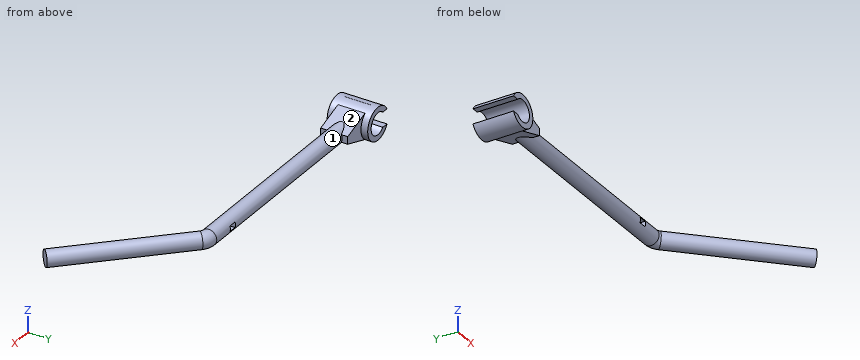
```python
from build123d import *

# Parameters (mm, degrees)
F0_R      = 6
F0_R_2    = 4
F1_DEPTH  = 7.5
F3_R      = 2.95
F4_DEPTH  = 80
F5_W      = 20
F5_H      = 5.5
F6_DEPTH  = 25
F12_DEPTH = 5
F13_W     = 3
F13_H     = 2
F14_DEPTH = 12.5
F16_R     = 2.95


with BuildPart() as f1:
    # F0 (on Front) → F1 (new body, symmetric)
    with BuildSketch(Plane.XZ):
        Circle(F0_R)
        Circle(F0_R_2, mode=Mode.SUBTRACT)
    extrude(amount=F1_DEPTH, both=True)

    # F3 (on offset) → F4 (join)
    with BuildSketch(Plane.YZ.offset(4.5)):
        Circle(F3_R)
    extrude(amount=F4_DEPTH)

    # F5 (on face) → F6 (cut)
    with BuildSketch(Plane.XZ.offset(7.5)):
        with Locations((-10, 0)):
            Rectangle(F5_W, F5_H)
    extrude(amount=-F6_DEPTH, mode=Mode.SUBTRACT)

    # F11 (on face) → F12 (join, symmetric)
    with BuildSketch(Plane.XZ):
        Polygon((13.7702096254, 1.3738754205), (0, 6.0186968185), (5.8568101376, 0), (0, -5.9087458067), (13.7702096254, -1.3786113122), align=None)
    extrude(amount=F12_DEPTH, both=True)

    # F13 (on Front) → F14 (cut, symmetric)
    with BuildSketch(Plane.XZ):
        with Locations((78, 0)):
            Rectangle(F13_W, F13_H)
    extrude(amount=F14_DEPTH, both=True, mode=Mode.SUBTRACT)

    # F17: sweep along a path in F15
    with BuildLine(Plane.XY) as f17_path:
        Line((84.5, 0), (87.5, 0))
        ThreePointArc((87.5, 0), (89.0307337295, -0.30448187), (90.3284271247, -1.1715728753))
        Line((90.3284271247, -1.1715728753), (125.6837661841, -36.5269119346))
    # F16 (on face) → F17 (sweep)
    with BuildSketch(Plane.YZ.offset(84.5)):
        Circle(F16_R)
    sweep(path=f17_path.line)


solid = f1.part
```
The model under review builds one solid part; all positions refer to its coordinate system, in mm. Face numbers are marked on the shaded views. A direction names the side the tool comes from. Give positions to 0.01 mm unless a question says otherwise; leave off trailing zeros. Write each loop counter-clockwise with the first axis right and the second up, starting at its lowest first coordinate (ties: lowest second). Pieces come first, ordered by that corner, then holes. Notation, with made-up numbers: (57, 89) -> (65, 89) arc R17 ccw to (65, 97) -> close; hole circle Ø2 at (83.5, 4.25). An arc over 180 degrees is marked (long way). Put each result on its own line as item: value.
(1) For pin 1 Ø4 at (x, z) = (102, -3.5) entering from +Y; pin 2 Ø0.7 at (x, y) = (-4, 0) entering from -Z; pin 3 Ø4 at (x, y) = (89.5, -1) entering from -Z, all flat-tipped, find the tip position at first contact; note any pin that passes through.
Results are:
pin 1: y = -8.45
pin 2: z = -4.76
pin 3: z = -2.95
(2) We need section A-A, the plane x = 45.5. Give the boundary of the cut face in (y, z), and give its area (3 significant figures).
Results are:
outline: circle Ø5.9 at (0, 0)
area: 27.3 mm²
(3) Tool access review of the marked faces 1 and 2: name each direction out of +Z, -Z, +X, -X, +Y, -Y from which nothing blocks a thin tool from reaching the whole face with its end or side.
Results are:
face 1: none
face 2: +Z
(4) To check wall thickness, follow probe 1 along Y at (x, z) = (11, 1); probe 2 along Y at (x, z) = (48, 0); probe 3 along X at (y, z) = (4.75, 0). State the ranges of each line that lie inside material, in increasing order. Write a range as from..to.
Results are:
probe 1: -5..5
probe 2: -2.95..2.95
probe 3: 4..13.77
